Part print with two shaded views. Sizes in mm from the minimum x, y, z corner. A direction names the side the tool comes from. Give positions to 0.01 mm unless a question says otherwise; leave off trailing zeros. Loops run counter-clockwise (first coordinate to the right, second up) from the corner with the lowest first, then second, coordinate; pieces in that order, holes last. Notation, with made-up numbers: (10.25, 16.5) -> (55.25, 16.5) arc R25 ccw to (55.25, 48.5) -> close; hole circle Ø1 at (-26.75, -40). An arc over 180 degrees is marked (long way). One line per question, with ' | ' between items.
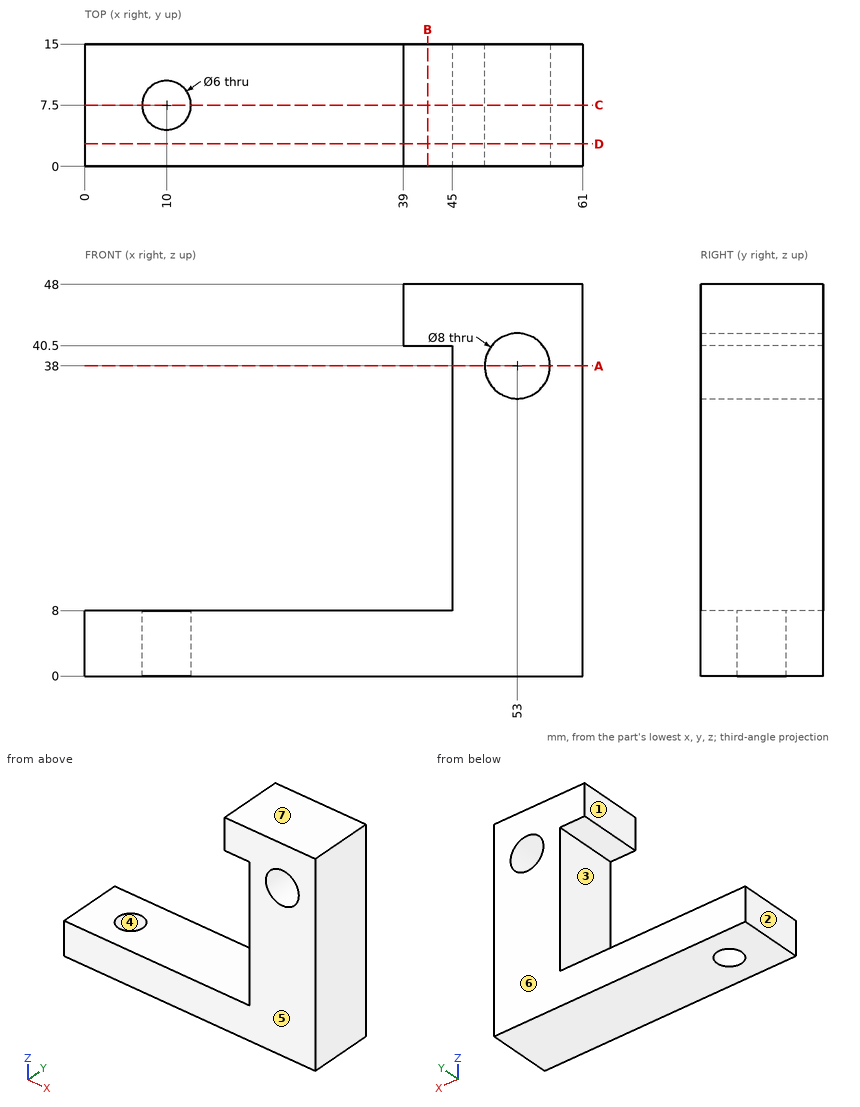
1) Drill centre lines: line 1 (X direction, y = 4.75, z = 31); line 2 (Z direction, x = 8, y = 14); line 3 (X direction, y = 2.75, z = 43). Where is each one in solid material? Low to high.
Found:
line 1: 45 to 61 | line 2: 0 to 8 | line 3: 39 to 61
2) Saw through at B-B (x = 42). Give the cut face in (y, z), and give its area (4 significant figures).
Found:
outline: (0, 0) -> (15, 0) -> (15, 8) -> (0, 8) -> close; (0, 40.5) -> (15, 40.5) -> (15, 48) -> (0, 48) -> close | area: 232.5 mm2
3) Saw through at C-C (y = 7.5). Give the cut face in (x, z), and give its area (3 significant figures).
Found:
outline: (0, 0) -> (7, 0) -> (7, 8) -> (0, 8) -> close; (13, 0) -> (61, 0) -> (61, 48) -> (39, 48) -> (39, 40.5) -> (45, 40.5) -> (45, 8) -> (13, 8) -> close; hole circle Ø8 at (53, 38) | area: 1,070 mm2
4) Pull direction Y, two halves, no side cores. Call the marked faces 4, 5, 6 and 7: pulls with the +Y half, pulls with the -Y half, needs draft (parallel to the pull), parting line crosses it, or undercut.
Found:
face 4: undercut | face 5: pulls with the -Y half | face 6: pulls with the +Y half | face 7: needs draft
5) Pin check, flat tips, straight feed: P1, Ø4.5, axis at y = 6.5, z = 22.5, coming from the -X side; P2, Ø5.5, axis at x = 10, y = 7.5, coming from the -Z side; P3, Ø6, axis at y = 5.5, z = 43.5, coming from the -X side. Stop position of each tip, or through.
Found:
P1: x = 45 | P2: through | P3: x = 39
6) Saw through at D-D (y = 2.75). Give the cut face in (x, z), and give its area (3 significant figures).
Found:
outline: (0, 0) -> (61, 0) -> (61, 48) -> (39, 48) -> (39, 40.5) -> (45, 40.5) -> (45, 8) -> (0, 8) -> close; hole circle Ø8 at (53, 38) | area: 1,120 mm2
7) Tool access for the marked faces 1, 2 and 3: list every direction of +Z, -Z, +X, -X, +Y, -Y with a clear straight run to the whole face (end or side of a thin tool).
Found:
face 1: +Z, -X, +Y, -Y | face 2: +Z, -Z, -X, +Y, -Y | face 3: -X, +Y, -Y
8) Saw through at A-A (z = 38). Give the cut face in (x, y).
Found:
outline: (45, 0) -> (49, 0) -> (49, 15) -> (45, 15) -> close; (57, 0) -> (61, 0) -> (61, 15) -> (57, 15) -> close
